```python
from build123d import *

# Parameters (mm, degrees)
IZIM1_W               = 50
IZIM1_H               = 180
TABAN_FLAN_1_DEPTH    = 10
RADYUS1_R             = 10
IZIM2_R               = 5.25
KES_EKSTR_ZYON1_DEPTH = 20


# Sheet-metal steps are written as plain solids
with BuildPart() as part:
    # Çizim1 → Taban-Flanş1 (new body)
    with BuildSketch(Plane.XY):
        Rectangle(IZIM1_W, IZIM1_H)
    extrude(amount=-TABAN_FLAN_1_DEPTH)

    # Radyus1
    radyus1_edges = [part.edges().sort_by_distance(p)[0] for p in [
        (25, -90, -5),
        (-25, -90, -5),
        (-25, 90, -5),
        (25, 90, -5),
    ]]
    fillet(radyus1_edges, radius=RADYUS1_R)

    # Çizim2 → Kes-Ekstrüzyon1 (cut)
    with BuildSketch(Plane.XY):
        with Locations((0, 70)):
            Circle(IZIM2_R)
        with Locations((0, -70)):
            Circle(IZIM2_R)
    extrude(amount=-KES_EKSTR_ZYON1_DEPTH, mode=Mode.SUBTRACT)


solid = part.part
```
Design review of the part built by this model. Coordinates are the model's own, in mm. Coordinates: 2 decimals unless noted, no trailing zeros. Write each loop counter-clockwise with the first axis right and the second up, starting at its lowest first coordinate (ties: lowest second). Pieces come first, ordered by that corner, then holes.
1) Add section C-C (x = 0). Write out the cut boundary in (y, z), plus the area to 3 significant figures.
2) Mouldability with a two-part tool opening along X and no side actions: class faces 1 (the flat face through (25, -1, -5)), 2 (the cylindrical face through (-1.138, -75.125, -4.93)), 3 (the flat face through (0, 90, -5)) as +X half, -X half, draft (parallel to the pull), parting line (faces both ways), or undercut.
3) Add section B-B (z = -4). Write out the cut boundary in (x, y), plus the area to 3 significant figures.
4) Add section D-D (x = 22). Write out the cut boundary in (y, z).
5) To check wall thickness, follow L1, parallel to Y at x = 0, z = -3.75; L2, parallel to Y at x = 3, z = -1; L3, parallel to X at y = -67, z = -6.75. State the ranges of each line that lie inside material, in increasing order.
6) Add section A-A (y = 70). Write out the cut boundary in (x, z), plus the area to 3 significant figures.
Check result:
1. outline: (-90, -10) - (-75.25, -10) - (-75.25, 0) - (-90, 0) - close; (-64.75, -10) - (64.75, -10) - (64.75, 0) - (-64.75, 0) - close; (75.25, -10) - (90, -10) - (90, 0) - (75.25, 0) - close
1. area: 1,590 mm2
2. face 1: +X half
2. face 2: undercut
2. face 3: draft
3. outline: (-25, -80) arc R10 ccw to (-15, -90) - (15, -90) arc R10 ccw to (25, -80) - (25, 80) arc R10 ccw to (15, 90) - (-15, 90) arc R10 ccw to (-25, 80) - close; hole circle Ø10.5 at (0, -70); hole circle Ø10.5 at (0, 70)
3. area: 8,740 mm2
4. outline: (-87.14, -10) - (87.14, -10) - (87.14, 0) - (-87.14, 0) - close
5. L1: y = -90 to -75.25, -64.75 to 64.75, 75.25 to 90
5. L2: y = -90 to -74.31, -65.69 to 65.69, 74.31 to 90
5. L3: x = -25 to -4.31, 4.31 to 25
6. outline: (-25, -10) - (-5.25, -10) - (-5.25, 0) - (-25, 0) - close; (5.25, -10) - (25, -10) - (25, 0) - (5.25, 0) - close
6. area: 395 mm2
